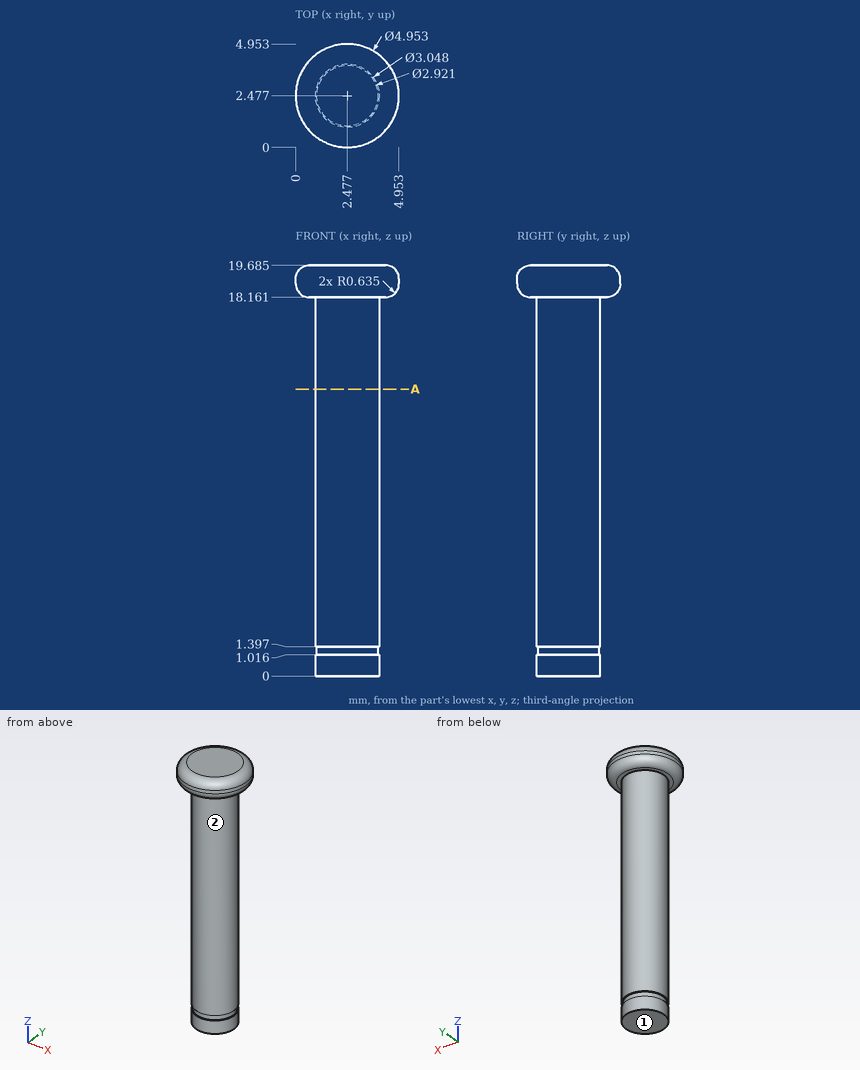
Could you check a few things on this drawing? It's one solid part, dimensions in mm from its lowest x, y, z. A direction names the side the tool comes from. Round coordinates to 2 decimals unless told otherwise and drop trailing zeros. Loops run counter-clockwise (first coordinate to the right, second up) from the corner with the lowest first, then second, coordinate; pieces in that order, holes last. Notation, with made-up numbers: (56.5, 25.5) -> (73.5, 25.5) arc R35 cw to (73.5, 63.5) -> close; hole circle Ø2 at (32, 57.5). An arc over 180 degrees is marked (long way). Answer as CSV lines item,"result".
1. For pin 1 (1 mm diameter, centred on x = 4, z = 2, fed in from -Y); pin 2 (2 mm diameter, centred on x = 2, z = 11.5, fed in from -Y); pin 3 (2 mm diameter, centred on y = 3, z = 3, fed in from -X), each with a flat end and sliding along its axis, tell me the tip position at first contact or that it passes through.
Final values:
pin 1,"stops at y = 1.35"
pin 2,"stops at y = 0.95"
pin 3,"stops at x = 0.95"
2. If we section it at A-A on z = 13.75: Please give me the cut outline in (x, y) (1 decimal).
Final values:
outline,"circle Ø3 at (2.5, 2.5)"
3. Which directions (+Z, -Z, +X, -X, +Y, -Y) give clear straight access to the entire face, cutting with the end or side of a thin tool? Please do the marked faces 1 and 2.
Final values:
face 1,"-Z, +X, -X, +Y, -Y"
face 2,"-Z"
4. If I drill on L1, parallel to Y at x = 2.55, z = 11.5 (1 decimal); L2, parallel to Y at x = 2.9, z = 11; L3, parallel to Z at x = 1.35, y = 1.35 (1 decimal), over which ranges is the centre line in solid material (lowest first)?
Final values:
L1,"y = 1 to 4"
L2,"y = 1.01 to 3.94"
L3,"z = 18.2 to 19.7"
